Verification items for the finished model (mm, model axes). A direction names the side the tool comes from. Round coordinates to 2 decimals unless told otherwise and drop trailing zeros. Write each loop counter-clockwise with the first axis right and the second up, starting at its lowest first coordinate (ties: lowest second). Pieces come first, ordered by that corner, then holes. Notation, with made-up numbers: M 74,-26.75 L 130,-26.75 A23 cw 130,12.25 Z; hole C 17,7 d7. An arc over 180 degrees is marked long. Answer in a Markdown table with one row per item. Add a question column.
1. Draft check along X on faces 4 (the flat face through (11, 7.366, 34)), 5 (the flat face through (-5, -5.715, 28)), 6 (the cylindrical face through (37.194, -0.876, 8.259)). Enter one of: pulls with the +X half, pulls with the -X half, needs draft (parallel to the pull), parting line crosses it, or undercut.
2. Sectioned sample at D-D on x = -27.94. Record the cut outline in (y, z) (1 decimal), plus the area to 3 significant figures.
3. Go/stop test with flat-tipped pins: pin 1 Ø1 at (x, z) = (14, 24.5) entering from -Y (3 decimals); pin 2 Ø4 at (y, z) = (-1.5, -22) entering from -X; pin 3 Ø4 at (y, z) = (-2.5, 21.5) entering from -X. Record where each tip stops, or that it passes through.
4. Material ranges on probe 1 along X at (y, z) = (5.25, 0); probe 2 along X at (y, z) = (-7, 0); probe 3 along X at (y, z) = (4.5, -14.5), recorded low to high.
5. Sectioned sample at C-C on z = 15. Record the cut outline in (x, y).
6. Set-up check for faces 1 (the cylindrical face through (14.994, -7.325, -24.062)), 2 (the flat face through (28.575, -4, -1)), 3 (the cylindrical face through (30.976, 5.801, -4.067)): record each of +Z, -Z, +X, -X, +Y, -Y from which the full face is reachable in a straight line by a thin tool's end or side.
```python
from build123d import *

# Parameters (mm, degrees)
SKETCH2_R          = 1.7272
CUT_EXTRUDE1_DEPTH = 55.61
SKETCH3_R          = 35.433
SKETCH3_R_2        = 31.242
CUT_EXTRUDE2_DEPTH = 3.175
SKETCH4_R          = 1.03251
CUT_EXTRUDE3_DEPTH = 3.175
CIRPATTERN1_COUNT  = 9
SKETCH5_R          = 3.175
CUT_EXTRUDE4_DEPTH = 9.525


with BuildPart() as part:
    # Sketch1 → Revolve1 (revolve)
    with BuildSketch(Plane.XY, mode=Mode.PRIVATE) as revolve1_sk:
        with BuildLine():
            Line((3.8608, 7.366), (38.1, 7.366))
            Line((38.1, 7.366), (38.1, -8.89))
            Line((38.1, -8.89), (22.6695, -8.89))
            Line((22.6695, -8.89), (22.6695, -7.874))
            Line((22.6695, -7.874), (21.1455, -7.874))
            Line((21.1455, -7.874), (21.1455, -8.89))
            Line((21.1455, -8.89), (10.9855, -8.89))
            Line((10.9855, -8.89), (10.9855, -6.391948453))
            ThreePointArc((10.9855, -6.391948453), (10.570616467, -5.000733157), (9.4615, -4.064))
            Line((9.4615, -4.064), (3.8608, 0))
            Line((3.8608, 0), (3.8608, 7.366))
        make_face()
    revolve(revolve1_sk.sketch.rotate(Axis((0, 101.60464546, 0), (0, 1, 0)), 90), axis=Axis((0, 101.60464546, 0), (0, 1, 0)))

    # Sketch2 → Cut-Extrude1 (cut, through all)
    with BuildSketch(Plane(origin=(0, 0, 0), x_dir=(0, 0, -1), z_dir=(1, 0, 0))):
        with Locations(Location((0, -2.286, 0), (0, 0, 270))):
            Circle(SKETCH2_R)
    extrude(amount=CUT_EXTRUDE1_DEPTH, mode=Mode.SUBTRACT)

    # Sketch3 → Cut-Extrude2 (cut)
    with BuildSketch(Plane(origin=(0, 7.366, 0), x_dir=(1, 0, 0), z_dir=(0, 1, 0))):
        with Locations(Location((0, 0, 0), (0, 0, 270))):
            Circle(SKETCH3_R)
        with Locations(Location((0, 0, 0), (0, 0, 270))):
            Circle(SKETCH3_R_2, mode=Mode.SUBTRACT)
    extrude(amount=-CUT_EXTRUDE2_DEPTH, mode=Mode.SUBTRACT)

    # Sketch4 → Cut-Extrude3 (cut)
    with BuildSketch(Plane(origin=(0, -8.89, 0), x_dir=(-1, 0, 0), z_dir=(0, -1, 0))):
        with Locations(Location((-13.97, 24.196749782, 0), (0, 0, 90))):
            Circle(SKETCH4_R)
    cut_extrude3 = extrude(amount=-CUT_EXTRUDE3_DEPTH, mode=Mode.SUBTRACT)

    # CirPattern1: Cut-Extrude3 ×9 about axis
    cirpattern1_axis = Axis((0, 0, 0), (0, 1, 0))
    for i in range(1, CIRPATTERN1_COUNT):
        add(cut_extrude3.rotate(cirpattern1_axis, i * 360 / CIRPATTERN1_COUNT), mode=Mode.SUBTRACT)

    # Sketch5 → Cut-Extrude4 (cut)
    with BuildSketch(Plane(origin=(38.1, 0, 0), x_dir=(0, 0, -1), z_dir=(1, 0, 0))):
        with Locations((0, -2.286)):
            Circle(SKETCH5_R)
    extrude(amount=-CUT_EXTRUDE4_DEPTH, mode=Mode.SUBTRACT)


solid = part.part
```
Geometry check:
| question | item | result |
|---|---|---|
| 1 | face 4 | needs draft |
| 1 | face 5 | undercut |
| 1 | face 6 | parting line crosses it |
| 2 | outline | M -8.9,-25.9 L 7.4,-25.9 L 7.4,-21.8 L 4.2,-21.8 L 4.2,-14 L 7.4,-14 L 7.4,14 L 4.2,14 L 4.2,21.8 L 7.4,21.8 L 7.4,25.9 L -8.9,25.9 L -8.9,1 L -5.7,1 L -5.7,-1 L -8.9,-1 Z |
| 2 | area | 786 mm2 |
| 3 | pin 1 | stops at y = -5.715 |
| 3 | pin 2 | stops at x = -32.43 |
| 3 | pin 3 | stops at x = -32.73 |
| 4 | probe 1 | x = -38.1 to -35.43, -31.24 to -3.86, 3.86 to 31.24, 35.43 to 38.1 |
| 4 | probe 2 | x = -38.1 to -28.97, -26.91 to -10.99, 10.99 to 38.1 |
| 4 | probe 3 | x = -35.23 to -32.33, -27.67 to 27.67, 32.33 to 35.23 |
| 5 | outline | M -35.02,-8.89 L -17,-8.89 L -17,-7.87 L -14.9,-7.87 L -14.9,-8.89 L 14.9,-8.89 L 14.9,-7.87 L 17,-7.87 L 17,-8.89 L 35.02,-8.89 L 35.02,7.37 L 32.1,7.37 L 32.1,4.19 L 27.41,4.19 L 27.41,7.37 L -27.41,7.37 L -27.41,4.19 L -32.1,4.19 L -32.1,7.37 L -35.02,7.37 Z |
| 6 | face 1 | -Y |
| 6 | face 2 | +X |
| 6 | face 3 | +Y |
